Here's how the part is built. I have some questions about the finished solid (model axes, mm). A direction names the side the tool comes from. Coordinates: 2 decimals unless noted, no trailing zeros. Write each loop counter-clockwise with the first axis right and the second up, starting at its lowest first coordinate (ties: lowest second). Pieces come first, ordered by that corner, then holes.
```python
from build123d import *

# Parameters (mm, degrees)
SKETCH1_R           = 9.525
BOSS_EXTRUDE1_DEPTH = 4.7625
SKETCH2_R           = 3.175
BOSS_EXTRUDE2_DEPTH = 4.7625
FILLET1_R           = 0.79248
BOSS_EXTRUDE3_START = 4.7625
SKETCH3_R           = 3.175
BOSS_EXTRUDE3_DEPTH = 4.7625
SKETCH13_R          = 2.97561
CUT_EXTRUDE1_DEPTH  = 17.497784


with BuildPart() as part:
    # Sketch1 → Boss-Extrude1 (new, symmetric)
    with BuildSketch(Plane(origin=(0, 0, 0), x_dir=(0, 0, -1), z_dir=(1, 0, 0))):
        with Locations(Location((0, 0, 0), (0, 0, 180))):
            Circle(SKETCH1_R)
    extrude(amount=BOSS_EXTRUDE1_DEPTH, both=True)

    # Sketch2 → Boss-Extrude2 (add)
    with BuildSketch(Plane(origin=(4.7625, 0, 0), x_dir=(0, 0, -1), z_dir=(1, 0, 0))):
        with Locations(Location((0, 0, 0), (0, 0, 180))):
            Circle(SKETCH2_R)
    extrude(amount=BOSS_EXTRUDE2_DEPTH)

    # Fillet1
    fillet1_edges = [part.edges().sort_by_distance(p)[0] for p in [
        (-4.7625, 0, -9.525),
        (4.7625, 0, -9.525),
    ]]
    fillet(fillet1_edges, radius=FILLET1_R)

    # Sketch3 → Boss-Extrude3 (add)
    with BuildSketch(Plane.ZY.offset(4.7625).offset(BOSS_EXTRUDE3_START)):
        Circle(SKETCH3_R)
    extrude(amount=-BOSS_EXTRUDE3_DEPTH)

    # Sketch13 → Cut-Extrude1 (cut, through all)
    with BuildSketch(Plane.XY):
        with Locations(Location((0, 0, 0), (0, 0, 180))):
            Circle(SKETCH13_R)
    extrude(amount=CUT_EXTRUDE1_DEPTH, mode=Mode.SUBTRACT)


solid = part.part
```
1) I need wall thicknesses on probe 1 along X at (y, z) = (1.5, 5); probe 2 along Y at (x, z) = (0, 5.5); probe 3 along X at (y, z) = (6.25, -4.5). Which ranges of each line are inside material? Lowest first, please.
Values follow:
probe 1: x = -4.76 to -2.57, 2.57 to 4.76
probe 2: y = -7.78 to -2.98, 2.98 to 7.78
probe 3: x = -4.76 to 4.76
2) We'd pull the mould along X, two halves only. Please class faces 1 (the face through (9.525, 0, 0)), 2 (the face through (-7.18, -3.1, -0.69)), 3 (the face through (0, 0, 0)): pulls with the +X half, pulls with the -X half, needs draft (parallel to the pull), parting line crosses it, or undercut.
Values follow:
face 1: pulls with the +X half
face 2: needs draft
face 3: undercut
3) Imagine slicing it at B-B on x = 8. Please give me the cut outline in (y, z) (3 decimals), then the cut area to 3 significant figures.
Values follow:
outline: circle Ø6.35 at (0, 0)
area: 31.7 mm2
4) Will these pins go through, and if not, where does the flat tip stop? pin 1 (3.5 mm diameter, centred on x = 0, y = 0, fed in from +Z); pin 2 (1.5 mm diameter, centred on x = -5, z = -2.5, fed in from -Y); pin 3 (3 mm diameter, centred on x = 7, y = 1.5, fed in from -Z) (3 decimals).
Values follow:
pin 1: stops at z = 0
pin 2: stops at y = -9.19
pin 3: stops at z = -3.175
5) On a 3-axis mill with a long thin cutter (end or side, diameter ignored), from which of +Z, -Z, +X, -X, +Y, -Y can I reach the whole of each face in a straight line? I mean faces 4 (the face through (-2.84, -0.89, 4.7)), 5 (the face through (0.056, 5.796, -7.559)), 6 (the face through (-4.762, 0, 4)), 7 (the face through (7.1, 2.8, 1.5)), 8 (the face through (-9.525, 0, 0)). Say none if no direction works.
Values follow:
face 4: +Z
face 5: +X, -X
face 6: -X
face 7: +X
face 8: +Z, -Z, -X, +Y, -Y
6) Imagine slicing it at C-C on x = 0. Please give me the cut outline in (y, z) (3 decimals).
Values follow:
outline: (-2.976, 0) - (-2.976, 9.048) arc R9.525 ccw (long way) to (2.976, 9.048) - (2.976, 0) - close
7) Imagine slicing it at A-A on y = 0. Please give me the cut outline in (x, z) (1 decimal).
Values follow:
outline: (-9.5, -3.2) - (-4.8, -3.2) - (-4.8, -8.7) arc R0.8 ccw to (-4, -9.5) - (4, -9.5) arc R0.8 ccw to (4.8, -8.7) - (4.8, -3.2) - (9.5, -3.2) - (9.5, 3.2) - (4.8, 3.2) - (4.8, 8.7) arc R0.8 ccw to (4, 9.5) - (3, 9.5) - (3, 0) - (-3, 0) - (-3, 9.5) - (-4, 9.5) arc R0.8 ccw to (-4.8, 8.7) - (-4.8, 3.2) - (-9.5, 3.2) - close
